Can you work these out from the drawing? Everything is in mm from the part's minimum corner. A direction names the side the tool comes from. Coordinates: 2 decimals unless noted, no trailing zeros. Order: outer loops, then holes, each group sorted by start corner. A loop starts at its lowest first (then second) coordinate and runs counter-clockwise, first axis right, second up. Notation, with made-up numbers: (-25, 19.25) -> (-1, 19.25) arc R17 cw to (-1, 24.25) -> close; hole circle Ø9 at (-20, 14.5). An arc over 180 degrees is marked (long way). Put each result on its own line as item: value. Start each with the question number.
Q1. If we section it at B-B (x = 23.25): Please give me the cut outline in (y, z), and give its area (4 significant figures).
Q2. We'd pull the mould along Y, two halves only. Please class the marked faces 4, 5 and 6: +Y half, -Y half, draft (parallel to the pull), parting line (faces both ways), or undercut.
Q3. If we section it at D-D (y = 11.5): Please give me the cut outline in (x, z), and give its area (3 significant figures).
Q4. If we section it at C-C (z = 23.5): Please give me the cut outline in (x, y).
Q5. If we section it at A-A (y = 2.5): Please give me the cut outline in (x, z).
Q6. Please list where these lines run through material, in increasing order: line 1 along Y through (x, z) = (15, 3.8); line 2 along X through (y, z) = (4.5, 21); line 3 along Z through (x, y) = (24.75, 17.5).
Q7. For the marked faces 1, 2 and 3, which set-ups out of +Z, -Z, +X, -X, +Y, -Y let a thin tool reach every point of the face, with its end or its side?
Q8. Will these pins go through, and if not, where does the flat tip stop? pin 1 (3.5 mm diameter, centred on x = 15, y = 11.5, fed in from +Z); pin 2 (5 mm diameter, centred on x = 25, z = 10.5, fed in from +Y).
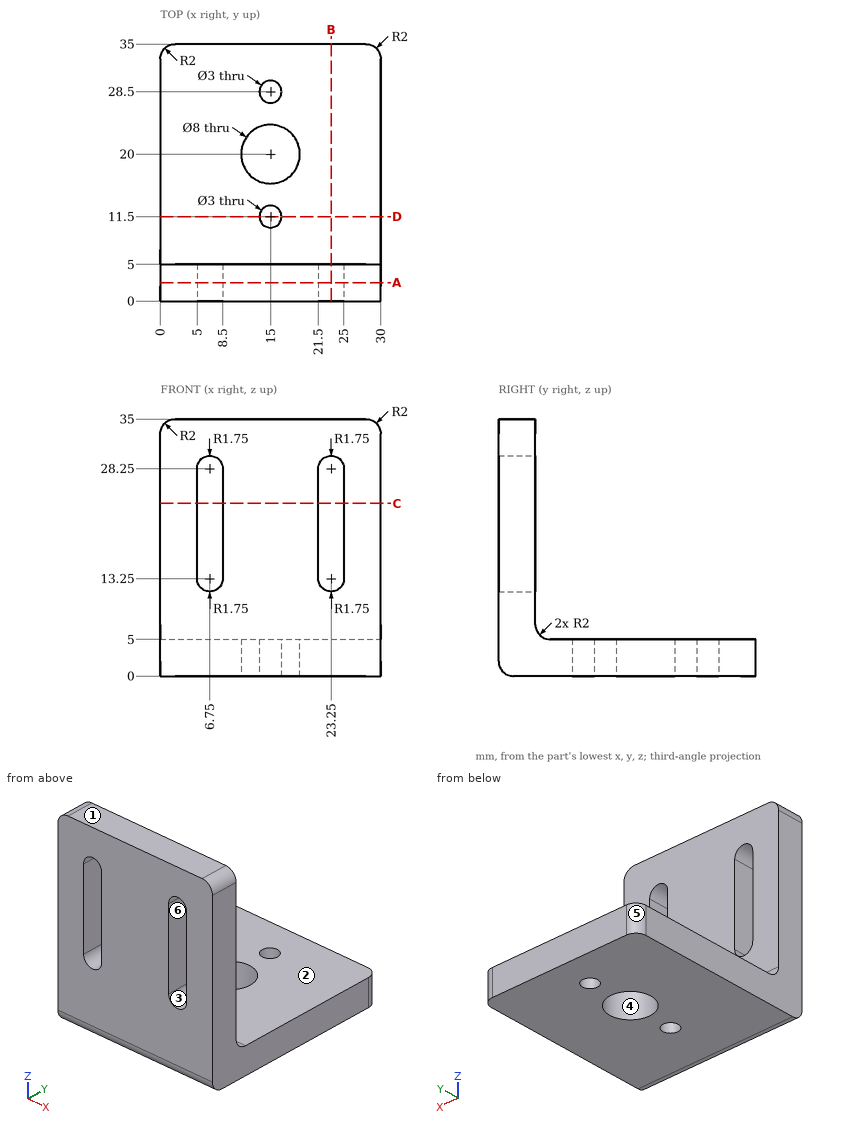
The answers:
1. outline: (0, 2) arc R2 ccw to (2, 0) -> (35, 0) -> (35, 5) -> (7, 5) arc R2 cw to (5, 7) -> (5, 11.5) -> (0, 11.5) -> close; (0, 30) -> (5, 30) -> (5, 35) -> (0, 35) -> close
1. area: 232.5 mm^2
2. face 4: undercut
2. face 5: +Y half
2. face 6: draft
3. outline: (0, 0) -> (13.5, 0) -> (13.5, 5) -> (0, 5) -> close; (16.5, 0) -> (30, 0) -> (30, 5) -> (16.5, 5) -> close
3. area: 135 mm^2
4. outline: (0, 0) -> (5, 0) -> (5, 5) -> (0, 5) -> close; (8.5, 0) -> (21.5, 0) -> (21.5, 5) -> (8.5, 5) -> close; (25, 0) -> (30, 0) -> (30, 5) -> (25, 5) -> close
5. outline: (0, 0) -> (30, 0) -> (30, 33) arc R2 ccw to (28, 35) -> (2, 35) arc R2 ccw to (0, 33) -> close; hole (5, 13.25) arc R1.75 ccw to (8.5, 13.25) -> (8.5, 28.25) arc R1.75 ccw to (5, 28.25) -> close; hole (21.5, 13.25) arc R1.75 ccw to (25, 13.25) -> (25, 28.25) arc R1.75 ccw to (21.5, 28.25) -> close
6. line 1: 0 to 10, 13 to 16, 24 to 27, 30 to 35
6. line 2: 0 to 5, 8.5 to 21.5, 25 to 30
6. line 3: 0 to 5
7. face 1: +Z, +X, -X, +Y, -Y
7. face 2: +Z, +X, -X, +Y
7. face 3: +Y, -Y
8. pin 1: z = 5
8. pin 2: y = 5
